Work out the finished part from the listing and answer in its coordinate system (mm). Round coordinates to 2 decimals unless told otherwise and drop trailing zeros. Loops run counter-clockwise (first coordinate to the right, second up) from the corner with the lowest first, then second, coordinate; pieces in that order, holes last. Notation, with made-up numbers: (41, 29) - (51, 29) arc R16 ccw to (51, 55) - close; hole circle Ø6 at (38, -16.75). An arc over 180 degrees is marked (long way). Answer as CSV lines item,"result". Start each with the question number.
```python
from build123d import *

# Parameters (mm, degrees)
SKETCH1_W           = 80
SKETCH1_H           = 400
BOSS_EXTRUDE1_DEPTH = 20
SKETCH4_R           = 32.5
CUT_EXTRUDE4_DEPTH  = 206.087962432
SKETCH6_R           = 25
CUT_EXTRUDE6_DEPTH  = 206.087962432


with BuildPart() as part:
    # Sketch1 → Boss-Extrude1 (new body)
    with BuildSketch(Plane.XY):
        Rectangle(SKETCH1_W, SKETCH1_H)
    extrude(amount=BOSS_EXTRUDE1_DEPTH)

    # Sketch4 → Cut-Extrude4 (cut, through all)
    with BuildSketch(Plane(origin=(0, 0.062016747, -0.8868808), x_dir=(1, 0, 0), z_dir=(0, -0.06975647374412192, 0.9975640502598245))):
        with Locations(Location((0, 120.405250769, 0), (0, 0, 90))):
            Circle(SKETCH4_R)
    extrude(amount=CUT_EXTRUDE4_DEPTH, mode=Mode.SUBTRACT)

    # Sketch6 → Cut-Extrude6 (cut, through all)
    with BuildSketch(Plane(origin=(0, 0.062016747, -0.8868808), x_dir=(1, 0, 0), z_dir=(0, -0.06975647374412192, 0.9975640502598246))):
        with Locations(Location((0, 120.405250769, 0), (0, 0, 270))):
            Circle(SKETCH6_R)
    extrude(amount=-CUT_EXTRUDE6_DEPTH, mode=Mode.SUBTRACT)


solid = part.part
```
Item 1: Determine the mould class of faces 1 (the face through (-1, 200, 10)), 2 (the face through (-1.429, 87.388, 10.918)), 3 (the face through (19.108, 136.833, 8.677)), 4 (the face through (-40, -3, 10)) for opening direction Y: pulls with the +Y half, pulls with the -Y half, needs draft (parallel to the pull), parting line crosses it, or undercut.
Item 2: Flat-ended cylindrical pins translate along their axes: pin 1 Ø5 at (x, y) = (-21.5, 130.5) entering from +Z; pin 2 Ø8 at (x, y) = (6, 69) entering from -Z; pin 3 Ø8 at (x, y) = (13.5, 131) entering from -Z. Find the tip coordinate at first contact, or state that the pin passes through.
Item 3: Find the intervals of material crossed by L1, parallel to Y at x = -11, z = 3.75; L2, parallel to Y at x = -7, z = 19.25; L3, parallel to X at y = 115.5, z = 1.75, in increasing order.
Item 4: Section A-A, the plane x = -20 is taken. Give the vertices of the cut face in (y, z).
Answer:
1,face 1,"pulls with the +Y half"
1,face 2,"undercut"
1,face 3,"undercut"
1,face 4,"needs draft"
2,pin 1,"stops at z = 8.41"
2,pin 2,"stops at z = 0"
2,pin 3,"passes through"
3,L1,"y = -200 to 97.93, 142.94 to 200"
3,L2,"y = -200 to 87.54, 151.17 to 200"
3,L3,"x = -40 to -24.48, 24.48 to 40"
4,outline,"(-200, 0) - (105.66, 0) - (105.21, 6.47) - (94.62, 5.73) - (93.62, 20) - (-200, 20) - close; (135.14, 8.56) - (135.74, 0) - (200, 0) - (200, 20) - (144.98, 20) - (145.73, 9.3) - close"
